Geometry check sheet. Reference: the model listing, model coordinates, mm. Coordinates: 2 decimals unless noted, no trailing zeros. Write each loop counter-clockwise with the first axis right and the second up, starting at its lowest first coordinate (ties: lowest second). Pieces come first, ordered by that corner, then holes. Notation, with made-up numbers: (20, -28.75) -> (32, -28.75) arc R21 cw to (32, -19.75) -> close; hole circle Ø5 at (-7.5, 46). An arc over 180 degrees is marked (long way). Answer in a Markdown table with one row per item. Add a question column.
1. Cross-section at B-B on z = -157.65. Record the cut outline in (x, y), and give its area (3 significant figures).
2. Depth check by flat-ended pin: P1, Ø4, axis at x = 6, z = -102.5, coming from the -Y side; P2, Ø7.5, axis at y = 122.4, z = -111.5, coming from the -X side. Enter the tip coordinate at first touch or a pass-through.
3. Cross-section at A-A on y = 122.4. Record the cut outline in (x, z), and give its area (3 significant figures).
4. Mould release check, pull along Z, two halves, no side actions. Record for faces 1 (the flat face through (10, 122, -101)), 2 (the flat face through (5, 125, -205)), 3 (the cylindrical face through (4.93, 99.762, -62.899)): pulls with the +Z half, pulls with the -Z half, needs draft (parallel to the pull), parting line crosses it, or undercut.
5. Scan lines: L1, parallel to Y at x = 3.25, z = -111.5; L2, parallel to Z at x = 5, y = 93.85; L3, parallel to Z at x = 8.5, y = 95.5. Record each from-to range of solid material in increasing order. Write a range as from..to.
Autodesk Inventor part; units mm, degrees
ref_plane "YZ Plane" through (0, 0, 0) normal (1, 0, 0) x (0, 1, 0)
ref_plane "XZ Plane" through (0, 0, 0) normal (0, 1, 0) x (-1, 0, 0)
ref_plane "XY Plane" through (0, 0, 0) normal (0, 0, 1) x (1, 0, 0)
sketch "Sketch1" plane through (0, 0, 0) normal (1, 0, 0) x (0, 1, 0)
  line L0 (0, 0) -> (247, 0)
  line L1 (247, 0) -> (247, -205)
  line L2 (247, -205) -> (0, -205)
  line L3 (0, -205) -> (0, 0)
  circle A0 centre (93.85, -65.35) radius 6.4
  circle A1 centre (93.85, -157.65) radius 6.4
  line L4 (93.85, -65.35) -> (93.85, -157.65)
  circle A2 centre (122.4, -111.5) radius 6.4
  line L5 (122.4, -111.5) -> (116, -111.5)
  line L6 (116, -111.5) -> (210.35, -111.5)
  circle A3 centre (210.35, -111.5) radius 6.4
  point P0 (122.35, 111.5)
  dimension "d5" = 12.8
  dimension "d0" = 247
  dimension "d1" = 205
  dimension "d3" = 12.8
  dimension "d4" = 92.3
  dimension "d6" = 94.35
  dimension "d7" = 12.8
  dimension "d10" = 12.8
extrude "Extrusion1" add sketch "Sketch1" along normal blind 10
properties part number "bigwall"
Results found:
| question | item | result |
|---|---|---|
| 1 | outline | (0, 0) -> (10, 0) -> (10, 87.45) -> (0, 87.45) -> close; (0, 100.25) -> (10, 100.25) -> (10, 247) -> (0, 247) -> close |
| 1 | area | 2,340 mm^2 |
| 2 | P1 | stops at y = 0 |
| 2 | P2 | passes through |
| 3 | outline | (0, -205) -> (10, -205) -> (10, -117.9) -> (0, -117.9) -> close; (0, -105.1) -> (10, -105.1) -> (10, 0) -> (0, 0) -> close |
| 3 | area | 1,920 mm^2 |
| 4 | face 1 | needs draft |
| 4 | face 2 | pulls with the -Z half |
| 4 | face 3 | undercut |
| 5 | L1 | y = 0..116, 128.8..203.95, 216.75..247 |
| 5 | L2 | z = -205..-164.05, -151.25..-71.75, -58.95..0 |
| 5 | L3 | z = -205..-163.83, -151.47..-71.53, -59.17..0 |
